Here's how the part is built. I have some questions about the finished solid (model axes, mm). Face numbers are marked on the shaded views. A direction names the side the tool comes from. Give positions to 0.01 mm unless a question says otherwise; leave off trailing zeros. Write each loop counter-clockwise with the first axis right and the second up, starting at its lowest first coordinate (ties: lowest second). Pieces come first, ordered by that corner, then holes. Notation, with made-up numbers: (-9, 80.5) -> (5, 80.5) arc R17 ccw to (5, 109.5) -> close; hole circle Ø8 at (3, -12). An arc over 180 degrees is marked (long way). Return JSON: item names as keys, results as strings.
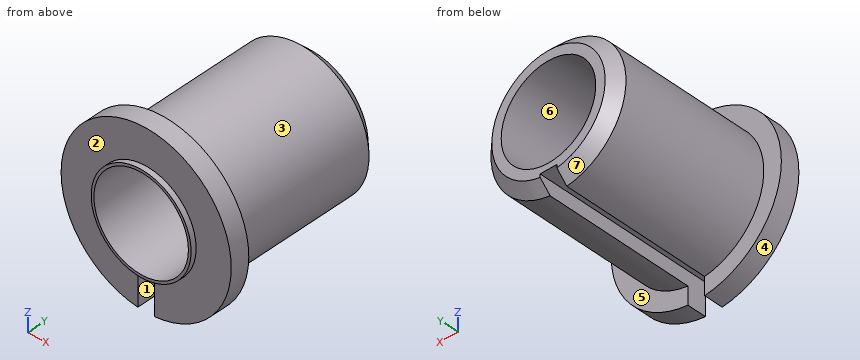
Autodesk Inventor part; units mm, degrees
ref_plane "1_XY" through (0, 7.112, 0) normal (0, 1, 0) x (1, 0, 0)
ref_plane "1_YZ" through (0, 7.112, 0) normal (1, 0, 0) x (0, 0, -1)
ref_plane "1_ZX" through (0, 7.112, 0) normal (0, 0, -1) x (0, 1, 0)
sketch "Sketch_1" plane through (0, 0, 0) normal (0, 0, 1) x (1, 0, 0)
  line L0 (-6.35, 0) -> (6.35, 0)
  arc A0 (6.35, 0) -> (6.096, 0.254) centre (6.096, 0) ccw
  line L1 (6.096, 0.254) -> (-6.096, 0.254)
  arc A1 (-6.096, 0.254) -> (-6.35, 0) centre (-6.096, 0) ccw
extrude "Extrusion1" add sketch "Sketch_1" along normal mid plane 13.0048
sketch "Sketch_6" plane through (0, 0, 0) normal (0, 0, 1) x (1, 0, 0)
  line L0 (0, 0.127) -> (0, 8.89)
  line L1 (0, 8.89) -> (2.667, 8.89)
  line L2 (2.667, 8.89) -> (3.175, 8.382)
  line L3 (3.175, 8.382) -> (3.175, 1.397)
  line L4 (3.175, 1.397) -> (4.0005, 1.397)
  line L5 (4.0005, 1.397) -> (4.0005, 0.508)
  line L6 (4.0005, 0.508) -> (2.3495, 0.508)
  line L7 (2.3495, 0.508) -> (2.3495, 0.127)
  line L8 (2.3495, 0.127) -> (0, 0.127)
  line L9 (0, 0.127) -> (0, 8.89)
revolve "Revolution1" add sketch "Sketch_6" angle 360 about axis through (0, 0.127, 0) along (0, -1, 0)
thread "Thread1"
sketch "Sketch_8" plane through (0, 0.254, 0) normal (0, 1, 0) x (1, 0, 0)
  line L0 (-0.3937, 2.4892) -> (0.3937, 2.4892)
  line L1 (0.3937, 2.4892) -> (0.3937, 10.4902)
  line L2 (0.3937, 10.4902) -> (-0.3937, 10.4902)
  line L3 (-0.3937, 10.4902) -> (-0.3937, 2.4892)
extrude "Extrusion2" cut sketch "Sketch_8" along normal blind 9.779
sketch "Sketch_10_ALT_Drilling_1" plane through (0, 0, 0) normal (0, 0, 1) x (1, 0, 0)
  line L0 (0, 0) -> (0, 9.525)
  line L1 (0, 9.525) -> (2.2225, 9.525)
  line L2 (2.2225, 9.525) -> (2.2225, 0)
  line L3 (2.2225, 0) -> (0, 0)
  line L4 (0, 0) -> (0, 9.525)
revolve "Revolution2" cut sketch "Sketch_10_ALT_Drilling_1" angle 360 about axis through (0, 0, 0) along (0, -1, 0)
sketch "Sketch_2" plane through (0, 0, 0) normal (0, 0, 1) x (1, 0, 0)
  line L0 (-6.35, 0.254) -> (-6.35, 0)
  line L1 (-6.35, 0) -> (6.35, 0)
  line L2 (6.35, 0) -> (6.35, 0.254)
  line L3 (6.35, 0.254) -> (-6.35, 0.254)
extrude "Extrusion3" cut sketch "Sketch_2" along normal mid plane 13.0048
ref_plane "1_XY" through (0, 7.112, 0) normal (0, 1, 0) x (1, 0, 0)
ref_plane "1_YZ" through (0, 7.112, 0) normal (1, 0, 0) x (0, 0, -1)
ref_plane "1_ZX" through (0, 7.112, 0) normal (0, 0, -1) x (0, 1, 0)
ref_plane "2_XY" through (0, 5.334, 0) normal (0, 1, 0) x (1, 0, 0)
ref_plane "2_YZ" through (0, 5.334, 0) normal (1, 0, 0) x (0, 0, -1)
ref_plane "2_ZX" through (0, 5.334, 0) normal (0, 0, -1) x (0, 1, 0)
ref_plane "3_XY" through (0, 3.556, 0) normal (0, 1, 0) x (1, 0, 0)
ref_plane "3_YZ" through (0, 3.556, 0) normal (1, 0, 0) x (0, 0, -1)
ref_plane "3_ZX" through (0, 3.556, 0) normal (0, 0, -1) x (0, 1, 0)
ref_plane "4_XY" through (0, 2.2225, 0) normal (0, 1, 0) x (1, 0, 0)
ref_plane "4_YZ" through (0, 2.2225, 0) normal (1, 0, 0) x (0, 0, -1)
ref_plane "4_ZX" through (0, 2.2225, 0) normal (0, 0, -1) x (0, 1, 0)
ref_plane "to_base_XY" through (0, 0, 0) normal (0, 1, 0) x (1, 0, 0)
ref_plane "to_base_YZ" through (0, 0, 0) normal (1, 0, 0) x (0, 0, -1)
ref_plane "to_base_ZX" through (0, 0, 0) normal (0, 0, -1) x (0, 1, 0)
properties part number "M20ANG2S1M202BR-bushing"
1. Suppose I cut it at D-D, the plane z = 3.5. List the corners of the cut face in (x, y) for me.
Taken from the geometry:
{"outline": "(-1.94, 0.51) -> (1.94, 0.51) -> (1.94, 1.4) -> (-1.94, 1.4) -> close"}
2. Which directions (+Z, -Z, +X, -X, +Y, -Y) give clear straight access to the entire face, cutting with the end or side of a thin tool? Please do the marked faces 1, 2, 3 and 4.
Taken from the geometry:
{"face 1": "-Z, +Y, -Y", "face 2": "-Y", "face 3": "+Y", "face 4": "+Y, -Y"}
3. For pin 1 Ø2.5 at (x, z) = (-2, 1.5) entering from -Y; pin 2 Ø1 at (y, z) = (7.5, -2.5) entering from -X; pin 3 Ø2 at (x, y) = (1, 8) entering from +Z (3 decimals); pin 4 Ø0.6 at (x, y) = (0, 5.5) entering from -Z, each with a flat end and sliding along its axis, tell me the tip position at first contact or that it passes through.
Taken from the geometry:
{"pin 1": "stops at y = 0.25", "pin 2": "stops at x = -2.47", "pin 3": "stops at z = 3.175", "pin 4": "stops at z = -2.49"}
4. If we mould it in two halves opening along X, with no side actions, what happens to the marked faces 5, 6 and 7? For each: released by +X, released by -X, zero draft, split by the parting line, or undercut.
Taken from the geometry:
{"face 5": "zero draft", "face 6": "undercut", "face 7": "split by the parting line"}
5. If I drill on line 1 (Z direction, x = 0, y = 1.25); line 2 (Z direction, x = 0, y = 4.25) (1 decimal); line 3 (X direction, y = 1.5, z = -2), over which ranges is the centre line in solid material (lowest first)? Write a range as [from, to].
Taken from the geometry:
{"line 1": "z = [-2.49, -2.22], [2.22, 4]", "line 2": "z = [-2.5, -2.2], [2.2, 3.2]", "line 3": "x = [-2.47, -0.97], [0.97, 2.47]"}
